from build123d import *

# Parameters (mm, degrees)
SKETCH1_R           = 6.477
BOSS_EXTRUDE3_DEPTH = 15.24
SKETCH4_R           = 4.064
CUT_EXTRUDE2_DEPTH  = 12.7
SKETCH5_R           = 2.539011159
CUT_EXTRUDE3_DEPTH  = 12.7


with BuildPart() as part:
    # Sketch1 → Boss-Extrude3 (new body)
    with BuildSketch(Plane(origin=(0, 0, 0), x_dir=(1, 0, 0), z_dir=(0, 1, 0))):
        with Locations(Location((0, 0, 0), (0, 0, 90))):
            Circle(SKETCH1_R)
    extrude(amount=BOSS_EXTRUDE3_DEPTH)

    # Sketch4 → Cut-Extrude2 (cut)
    with BuildSketch(Plane.XZ):
        with Locations(Location((0, 0, 0), (0, 0, 270))):
            Circle(SKETCH4_R)
    extrude(amount=-CUT_EXTRUDE2_DEPTH, mode=Mode.SUBTRACT)

    # Sketch5 → Cut-Extrude3 (cut)
    with BuildSketch(Plane.XZ.offset(-12.7)):
        with Locations(Location((0, 0, 0), (0, 0, 270))):
            Circle(SKETCH5_R)
    extrude(amount=-CUT_EXTRUDE3_DEPTH, mode=Mode.SUBTRACT)


solid = part.part
The model under review builds one solid part; all positions refer to its coordinate system, in mm. A direction names the side the tool comes from. Round coordinates to 2 decimals unless told otherwise and drop trailing zeros. Write each loop counter-clockwise with the first axis right and the second up, starting at its lowest first coordinate (ties: lowest second). Pieces come first, ordered by that corner, then holes. Notation, with made-up numbers: M 71.5,85 L 123.5,85 A26 ccw 123.5,108 Z; hole C 74,58.25 d2. An arc over 180 degrees is marked long. Answer as CSV lines item,"result". Start each with the question number.
Q1. Consider section B-B, the plane z = 0. Give the boundary of the cut face in (x, y), then the cut area to 3 significant figures.
Q2. Consider section C-C, the plane y = 11.5. Give the boundary of the cut face in (x, z).
Q3. Clearance check with a flat-ended pin moving along its axis: P1, Ø3, axis at y = 3, z = -3.5, coming from the -X side. State where the tip first meets the part, or that it passes through.
Q4. Consider section D-D, the plane x = 3.5. Give the boundary of the cut face in (y, z), then the cut area to 3 significant figures.
Q5. Consider section A-A, the plane x = 0. Give the boundary of the cut face in (y, z).
Q6. Tool access review of faces 4 (the face through (-2, 12.7, 2)), 5 (the face through (-3, 0, -3)): name each direction out of +Z, -Z, +X, -X, +Y, -Y from which nothing blocks a thin tool from reaching the whole face with its end or side.
Q7. The part is to be moulded in two halves that separate along Z. For faces 1 (the face through (6.323, 7.513, 1.404)), 2 (the face through (-3.967, 6.261, 0.881)), 3 (the face through (3, 15.24, 0)), say which applies: +Z half, -Z half, draft (parallel to the pull), parting line (faces both ways), or undercut.
Q8. Wall thickness on line 1 along X through (y, z) = (13.45, 0); line 2 along X through (y, z) = (7.75, 0); line 3 along Y through (x, z) = (1.5, 2.75): over which ranges is each line inside the solid? List them lowest first.
Result set:
1,outline,"M -6.48,0 L -4.06,0 L -4.06,12.7 L -2.54,12.7 L -2.54,15.24 L -6.48,15.24 Z; M 2.54,12.7 L 4.06,12.7 L 4.06,0 L 6.48,0 L 6.48,15.24 L 2.54,15.24 Z"
1,area,"81.3 mm²"
2,outline,"C 0,0 d12.95; hole C 0,0 d8.13"
3,P1,"stops at x = -6.16"
4,outline,"M 0,-5.45 L 15.24,-5.45 L 15.24,5.45 L 0,5.45 L 0,2.07 L 12.7,2.07 L 12.7,-2.07 L 0,-2.07 Z"
4,area,"114 mm²"
5,outline,"M 0,-6.48 L 15.24,-6.48 L 15.24,-2.54 L 12.7,-2.54 L 12.7,-4.06 L 0,-4.06 Z; M 0,4.06 L 12.7,4.06 L 12.7,2.54 L 15.24,2.54 L 15.24,6.48 L 0,6.48 Z"
6,face 4,"-Y"
6,face 5,"+Z, -Z, +X, -X, -Y"
7,face 1,"parting line"
7,face 2,"undercut"
7,face 3,"draft"
8,line 1,"x = -6.48 to -2.54, 2.54 to 6.48"
8,line 2,"x = -6.48 to -4.06, 4.06 to 6.48"
8,line 3,"y = 12.7 to 15.24"
